```python
from build123d import *

# Parameters (mm, degrees)
SKETCH1_W           = 20
SKETCH1_H           = 26
BOSS_EXTRUDE1_DEPTH = 12
SKETCH2_R           = 3.1
CUT_EXTRUDE1_DEPTH  = 40
SKETCH3_R           = 2.6
SKETCH3_R_2         = 1.5
CUT_EXTRUDE2_DEPTH  = 40


with BuildPart() as part:
    # Sketch1 → Boss-Extrude1 (new body)
    with BuildSketch(Plane.XY):
        with Locations((0, 13)):
            Rectangle(SKETCH1_W, SKETCH1_H)
    extrude(amount=BOSS_EXTRUDE1_DEPTH)

    # Sketch2 → Cut-Extrude1 (cut, symmetric)
    with BuildSketch(Plane.XY):
        with Locations((0, 19)):
            Circle(SKETCH2_R)
    extrude(amount=CUT_EXTRUDE1_DEPTH, both=True, mode=Mode.SUBTRACT)

    # Sketch3 → Cut-Extrude2 (cut, symmetric)
    with BuildSketch(Plane(origin=(0, 0, 0), x_dir=(1, 0, 0), z_dir=(0, 1, 0))):
        with Locations(Location((6.5, -6, 0), (0, 0, 270))):
            Circle(SKETCH3_R)
        with Locations(Location((0, -6, 0), (0, 0, 270))):
            Circle(SKETCH3_R_2)
    extrude(amount=CUT_EXTRUDE2_DEPTH, both=True, mode=Mode.SUBTRACT)


solid = part.part
```
Input: part model. Units: mm. Frame: model coordinates. Give positions to 0.01 mm unless a question says otherwise; leave off trailing zeros. Order: outer loops, then holes, each group sorted by start corner. A loop starts at its lowest first (then second) coordinate and runs counter-clockwise, first axis right, second up.
1. Cut plane C-C (z = 6). Return loops of the section in (x, y), and give its area (3 significant figures).
Computed:
outline: (-10, 0) - (-1.5, 0) - (-1.5, 16.29) arc R3.1 cw to (-1.5, 21.71) - (-1.5, 26) - (-10, 26) - close; (1.5, 0) - (3.9, 0) - (3.9, 26) - (1.5, 26) - (1.5, 21.71) arc R3.1 cw to (1.5, 16.29) - close; (9.1, 0) - (10, 0) - (10, 26) - (9.1, 26) - close
area: 294 mm2
2. Draft query along Z for faces 1 (the face through (0, 13, 0)), 2 (the face through (0.07, 8.26, 4.5)), 3 (the face through (-2, 0, 6)). Return one class per face: released by +Z, released by -Z, zero draft, split by the parting line, or undercut.
Computed:
face 1: released by -Z
face 2: undercut
face 3: zero draft
3. Pin query (flat end, axial travel): pin 1 Ø7 at (x, y) = (0, 19) entering from -Z; pin 2 Ø3 at (x, z) = (6.5, 6) entering from -Y. Return the tip coordinate at first contact, or that it passes through.
Computed:
pin 1: stops at z = 0
pin 2: passes through
4. Cut plane A-A (x = 6.5). Return loops of the section in (y, z).
Computed:
outline: (0, 0) - (26, 0) - (26, 3.4) - (0, 3.4) - close; (0, 8.6) - (26, 8.6) - (26, 12) - (0, 12) - close
5. Cut plane B-B (y = 16.75). Return loops of the section in (x, z), and give its area (3 significant figures).
Computed:
outline: (-10, 0) - (-2.13, 0) - (-2.13, 12) - (-10, 12) - close; (2.13, 0) - (10, 0) - (10, 12) - (2.13, 12) - close; hole circle Ø5.2 at (6.5, 6)
area: 168 mm2
6. Line query: probe 1 along Z at (x, y) = (0, 3.5); probe 2 along X at (y, z) = (16.5, 6); probe 3 along X at (y, z) = (6.75, 6). Output: solid intervals per line, ascending.
Computed:
probe 1: z = 0 to 4.5, 7.5 to 12
probe 2: x = -10 to -1.83, 1.83 to 3.9, 9.1 to 10
probe 3: x = -10 to -1.5, 1.5 to 3.9, 9.1 to 10
7. Cut plane D-D (x = 0). Return loops of the section in (y, z).
Computed:
outline: (0, 0) - (15.9, 0) - (15.9, 4.5) - (0, 4.5) - close; (0, 7.5) - (15.9, 7.5) - (15.9, 12) - (0, 12) - close; (22.1, 0) - (26, 0) - (26, 4.5) - (22.1, 4.5) - close; (22.1, 7.5) - (26, 7.5) - (26, 12) - (22.1, 12) - close
